Input: dimensioned drawing with shaded views. Units: mm. Origin: part minimum x, y, z. A direction names the side the tool comes from. Coordinates: 2 decimals unless noted, no trailing zeros. Loops run counter-clockwise (first coordinate to the right, second up) from the corner with the lowest first, then second, coordinate; pieces in that order, holes last. Notation, with made-up numbers: (88, 9.5) - (128, 9.5) arc R21 cw to (128, 39.5) - close; hole circle Ø3 at (-35.75, -11). An arc over 180 degrees is marked (long way). Put each result on its own line as item: value. Start each with the question number.
1) Section B-B on y = 50.8. Output: boundary loops of the cut face in (x, z) (1 decimal), and give its area (3 significant figures).
2) Material intervals for line 1 along X through (y, z) = (50, 43) (1 decimal); line 2 along Y through (x, z) = (38.1, 16.5); line 3 along Y through (x, z) = (38.1, 38), sorted ascending. Write a range as from..to.
3) Section D-D on x = 68. Output: boundary loops of the cut face in (y, z), and give its area (3 significant figures).
4) Draft query along X for the marked faces 1, 2, 3 and 4. Return one class per face: +X half, -X half, draft (parallel to the pull), parting line (faces both ways), or undercut.
5) Section A-A on x = 38.1. Output: boundary loops of the cut face in (y, z), and give its area (3 significant figures).
6) Contact query for flat-ended pins moving along their axis: pin 1 Ø14 at (x, y) = (36, 5) entering from -Z; pin 2 Ø8 at (y, z) = (41, 62.5) entering from +X; pin 3 Ø8 at (x, z) = (45, 18) entering from -Y. Output: stop coordinate, or through.
7) Reachability of the marked faces 5, 6 and 7 from +Z, -Z, +X, -X, +Y, -Y: full face, straight path, thin tool, end or side. Return the list, or none.
8) Section C-C on z = 38.1. Output: boundary loops of the cut face in (x, y) (1 decimal).
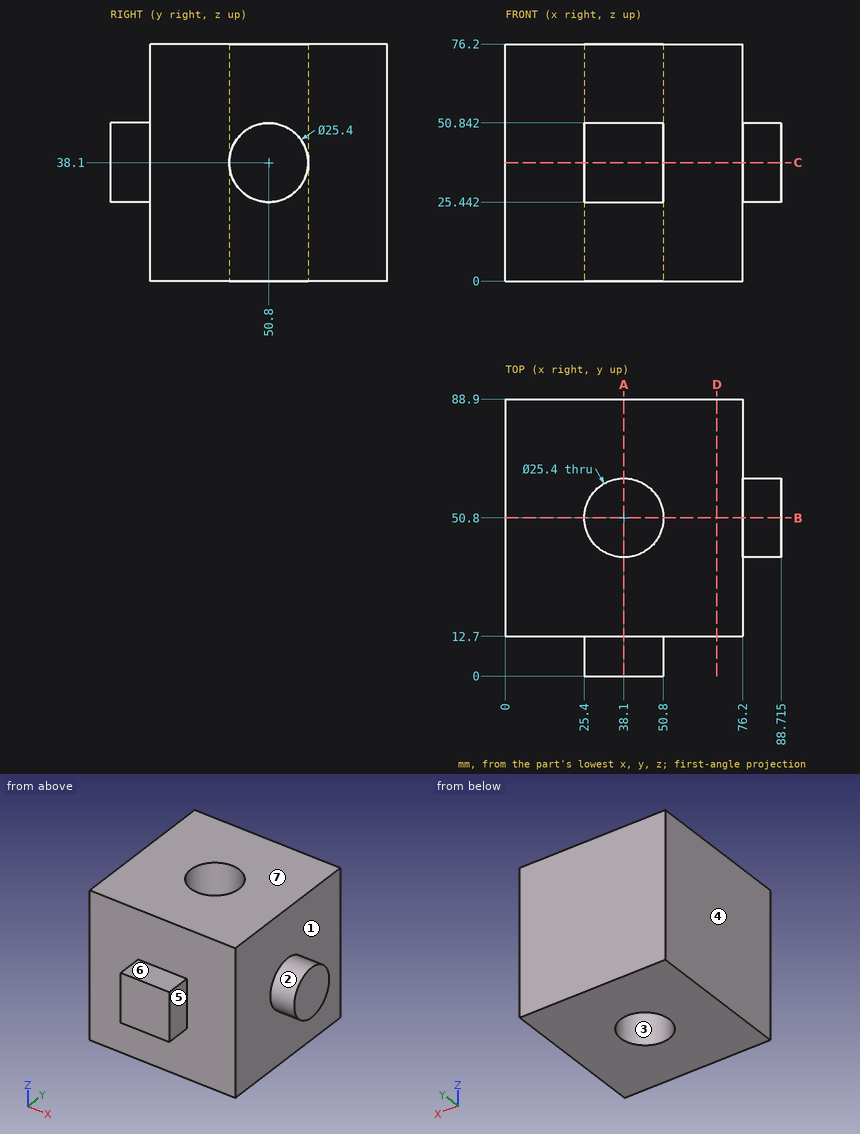
Answer block:
1. outline: (0, 0) - (25.4, 0) - (25.4, 76.2) - (0, 76.2) - close; (50.8, 0) - (76.2, 0) - (76.2, 25.4) - (88.7, 25.4) - (88.7, 50.8) - (76.2, 50.8) - (76.2, 76.2) - (50.8, 76.2) - close
1. area: 4,190 mm²
2. line 1: x = 0..25.4, 50.8..88.7
2. line 2: y = 12.7..38.1, 63.5..88.9
2. line 3: y = 0..38.1, 63.5..88.9
3. outline: (12.7, 0) - (88.9, 0) - (88.9, 76.2) - (12.7, 76.2) - close
3. area: 5,810 mm²
4. face 1: +X half
4. face 2: draft
4. face 3: undercut
4. face 4: -X half
5. outline: (0, 25.44) - (12.7, 25.44) - (12.7, 0) - (38.1, 0) - (38.1, 76.2) - (12.7, 76.2) - (12.7, 50.84) - (0, 50.84) - close; (63.5, 0) - (88.9, 0) - (88.9, 76.2) - (63.5, 76.2) - close
5. area: 4,190 mm²
6. pin 1: stops at z = 25.44
6. pin 2: stops at x = 76.2
6. pin 3: stops at y = 12.7
7. face 5: +Z, -Z, +X, -Y
7. face 6: +Z, +X, -X, -Y
7. face 7: +Z, +X, -X, +Y, -Y
8. outline: (0, 12.7) - (25.4, 12.7) - (25.4, 0) - (50.8, 0) - (50.8, 12.7) - (76.2, 12.7) - (76.2, 38.1) - (88.7, 38.1) - (88.7, 63.5) - (76.2, 63.5) - (76.2, 88.9) - (0, 88.9) - close; hole circle Ø25.4 at (38.1, 50.8)
